Here's the drawing with two shaded views (mm, measured from the low corner). I have some questions. A direction names the side the tool comes from. Coordinates: 2 decimals unless noted, no trailing zeros. Loops run counter-clockwise (first coordinate to the right, second up) from the corner with the lowest first, then second, coordinate; pieces in that order, holes last. Notation, with made-up numbers: M 62,-13 L 98,-13 A29 cw 98,21 Z; hole C 57.5,41.5 d7. An arc over 180 degrees is marked long. Return JSON: item names as keys, results as strings. Group by question number.
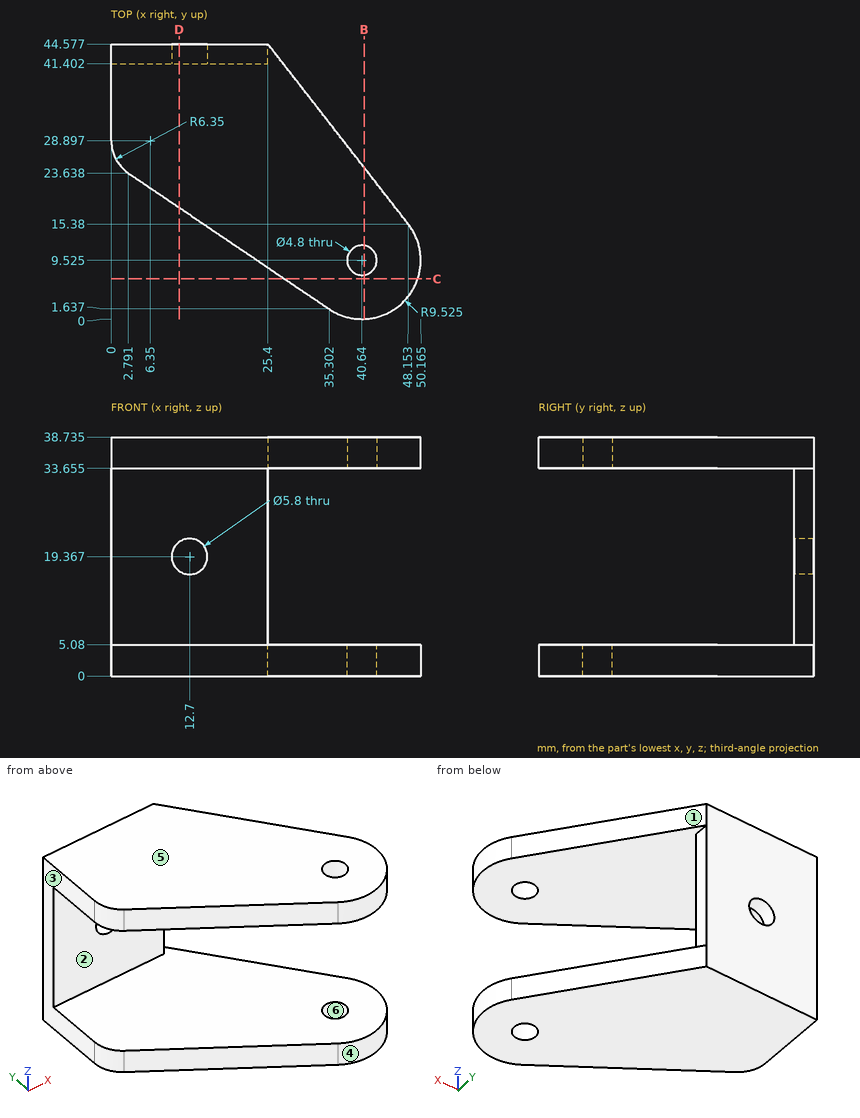
1) If I drill on line 1 (Z direction, x = 8.5, y = 39.5) (1 decimal); line 2 (Y direction, x = 40.64, z = 36.65) (1 decimal); line 3 (Z direction, x = 12, y = 42) (1 decimal), over which ranges is the centre line in solid material (lowest first)? Write a range as from..to.
2) For pin 1 (6 mm diameter, centred on y = 15.5, z = 6.5, fed in from -X); pin 2 (12.5 mm diameter, centred on x = 18, z = 18.5, fed in from -Y); pin 3 (6 mm diameter, centred on y = 27, z = 31.5, fed in from +X) (1 decimal), each with a flat end and sliding along its axis, tell me the tip position at first contact or that it passes through.
3) Suppose I cut it at D-D, the plane x = 11. List the corners of the cut face in (y, z) for me (1 decimal).
4) Suppose I cut it at B-B, the plane x = 41. List the corners of the cut face in (y, z) for me (1 decimal), then the cut area to 3 significant figures.
5) For the marked faces 1 and 2, which set-ups out of +Z, -Z, +X, -X, +Y, -Y let a thin tool reach every point of the face, with its end or its side?
6) Suppose I cut it at C-C, the plane y = 6.5. List the corners of the cut face in (x, z) for me (1 decimal).
7) If we mould it in two halves opening along X, with no side actions, what happens to the marked faces 3, 4, 5 and 6? For each: +X half, -X half, draft (parallel to the pull), parting line (faces both ways), or undercut.
Returned:
{
 "1": {"line 1": "z = 0..5.1, 33.7..38.7", "line 2": "y = 0..7.1, 11.9..25", "line 3": "z = 0..16.6, 22.2..38.7"},
 "2": {"pin 1": "stops at x = 10.91", "pin 2": "stops at y = 41.4", "pin 3": "stops at x = 40.7"},
 "3": {"outline": "M 18.1,0 L 44.6,0 L 44.6,17 L 41.4,17 L 41.4,5.1 L 18.1,5.1 Z; M 18.1,33.7 L 41.4,33.7 L 41.4,21.7 L 44.6,21.7 L 44.6,38.7 L 18.1,38.7 Z"},
 "4": {"outline": "M 0,0 L 7.2,0 L 7.2,5.1 L 0,5.1 Z; M 0,33.7 L 7.2,33.7 L 7.2,38.7 L 0,38.7 Z; M 11.9,0 L 24.6,0 L 24.6,5.1 L 11.9,5.1 Z; M 11.9,33.7 L 24.6,33.7 L 24.6,38.7 L 11.9,38.7 Z", "area": "201 mm²"},
 "5": {"face 1": "+Z, -Z, +X, +Y", "face 2": "+X, -X, -Y"},
 "6": {"outline": "M 28.1,0 L 49.7,0 L 49.7,5.1 L 28.1,5.1 Z; M 28.1,33.7 L 49.7,33.7 L 49.7,38.7 L 28.1,38.7 Z"},
 "7": {"face 3": "-X half", "face 4": "parting line", "face 5": "draft", "face 6": "undercut"}
}
